from build123d import *

# Parameters (mm, degrees)
SKETCH_R     = 2.1
PAD_DEPTH    = 3
SKETCH001_W  = 7.4
SKETCH001_H  = 7.4
POCKET_DEPTH = 5


with BuildPart() as pocket:
    # Sketch → Pad (new body)
    with BuildSketch(Plane.XY):
        with BuildLine():
            Line((0, 20), (65, 20))
            Line((65, 20), (65, 0))
            Line((20, 0), (65, 0))
            Line((20, -6), (20, 0))
            ThreePointArc((10, -6), (15, -11), (20, -6))
            Line((10, 0), (10, -6))
            Line((0, 0), (10, 0))
            Line((0, 0), (0, 20))
        make_face()
        with Locations((15, -6)):
            Circle(SKETCH_R, mode=Mode.SUBTRACT)
    extrude(amount=PAD_DEPTH)

    # Sketch001 → Pocket (cut)
    with BuildSketch(Plane(origin=(0, 0, 0), x_dir=(1, 0, 0), z_dir=(0, 0, -1))):
        with Locations((18.7, -10)):
            Rectangle(SKETCH001_W, SKETCH001_H)
        with Locations((46.1, -10)):
            Rectangle(SKETCH001_W, SKETCH001_H)
    extrude(amount=-POCKET_DEPTH, mode=Mode.SUBTRACT)


with BuildPart() as part_mirroring:
    # Part__Mirroring: instance of Pocket
    add(pocket.part.mirror(Plane(origin=(0, 0, 0), x_dir=(0, -1, 0), z_dir=(1, 0, 0))))


with BuildPart() as part_mirroring_1:
    # Part__Mirroring placement: moved
    add(part_mirroring.part.moved(Location((130, 0, 0))))


with BuildPart() as fusion:
    # Fusion base: copy of Pocket
    add(pocket.part)

    # Fusion: union Part__Mirroring
    add(part_mirroring_1.part)


solid = fusion.part
Build history of the part. All positions in model axes, mm. A direction names the side the tool comes from. Round coordinates to 2 decimals unless told otherwise and drop trailing zeros. Loops run counter-clockwise (first coordinate to the right, second up) from the corner with the lowest first, then second, coordinate; pieces in that order, holes last. Notation, with made-up numbers: (-34.75, 62.5) -> (16.25, 62.5) arc R18 cw to (16.25, 90.5) -> close; hole circle Ø4 at (75.25, 5). An arc over 180 degrees is marked (long way). One line per item, written item: value. Start each with the question number.
Q1. Two-plate mould, pull along Y, no slides. Class faces 5 (the face through (15, -11, 1)), 6 (the face through (110, -3, 1)), 7 (the face through (19, 13.7, 1)): released by +Y, released by -Y, zero draft, split by the parting line, or undercut.
Q2. Cut at B-B on z = 1.5. Count the separate pieces of the cut face and the enclosed holes in it, plus the area to 3 significant figures.
Q3. Cut at A-A on y = 10. List the corners of the cut face in (x, z).
Q4. Drop a flat-ended pin along its axis: pin 1 Ø1 at (y, z) = (-4, 1) entering from -X. Give the stop position or say it passes through.
Q5. Probe line 1 along X through (y, z) = (11, 0.75); line 2 along Y through (x, z) = (18, 2.85); line 3 along Y through (x, z) = (84, 1.7). List the from-to ranges inside material, lowest first.
Q6. Cut at C-C on x = 101. List the corners of the cut face in (y, z).
Q7. 3-axis set-ups, long thin cutter, end or side, ignore diameter. For faces 1 (the face through (20, -3, 1)), 2 (the face through (125, 0, 1)), 3 (the face through (0, 10, 1)), 4 (the face through (111, 13.7, 1)): which of +Z, -Z, +X, -X, +Y, -Y reach the whole face in a straight line?
Computed:
1. face 5: released by -Y
1. face 6: zero draft
1. face 7: undercut
2. separate pieces: 1
2. enclosed holes: 6
2. area: 2,550 mm²
3. outline: (0, 0) -> (15, 0) -> (15, 3) -> (0, 3) -> close; (22.4, 0) -> (42.4, 0) -> (42.4, 3) -> (22.4, 3) -> close; (49.8, 0) -> (80.2, 0) -> (80.2, 3) -> (49.8, 3) -> close; (87.6, 0) -> (107.6, 0) -> (107.6, 3) -> (87.6, 3) -> close; (115, 0) -> (130, 0) -> (130, 3) -> (115, 3) -> close
4. pin 1: x = 10
5. line 1: 0 to 15, 22.4 to 42.4, 49.8 to 80.2, 87.6 to 107.6, 115 to 130
5. line 2: -10 to 6.3, 13.7 to 20
5. line 3: 0 to 6.3, 13.7 to 20
6. outline: (0, 0) -> (20, 0) -> (20, 3) -> (0, 3) -> close
7. face 1: +Z, -Z, -Y
7. face 2: +Z, -Z, +X, -Y
7. face 3: +Z, -Z, -X, +Y, -Y
7. face 4: +Z, -Z
